For this review, take the finished solid that the model builds, in its own axes (mm). Face numbers are marked on the shaded views. A direction names the side the tool comes from. Give positions to 0.01 mm unless a question says otherwise; leave off trailing zeros. Order: outer loops, then holes, each group sorted by start corner. A loop starts at its lowest first (then second) coordinate and runs counter-clockwise, first axis right, second up. Notation, with made-up numbers: M -39,-32.75 L -16,-32.75 A14 cw -16,-5.75 Z; hole C 1,79 d9. An arc over 180 degrees is marked long. Use CSV: the item, a comma, the result in double quotes. Start each with the question number.
(1) Draft analysis for pull direction Y (two halves, no side actions). For the marked faces 1, 2 and 3, state which applies: pulls with the +Y half, pulls with the -Y half, needs draft (parallel to the pull), parting line crosses it, or undercut.
(2) Clearance check with flat-ended pins moving along their axes: P1, Ø1, axis at x = 2, z = 0.5, coming from the -Y side; P2, Ø4, axis at x = 0, y = 0, coming from the +Z side. State where each tip first meets the part, or that it passes through.
(3) Consider section C-C (z = 0.4). Write out the cut boundary in (x, y), and give its area (3 significant figures).
(4) Tool access review of the marked faces 4 and 5: name each direction out of +Z, -Z, +X, -X, +Y, -Y from which nothing blocks a thin tool from reaching the whole face with its end or side.
(5) Consider section D-D (z = 1.6). Write out the cut boundary in (x, y), and give its area (3 significant figures).
(6) Wall thickness on L1, parallel to Y at x = 0, z = 1; L2, parallel to Y at x = 0, z = 0.55; L3, parallel to Z at x = -1.25, y = -4: over which ranges is each line inside the solid? List them lowest first. Write a range as from..to.
(7) Consider section A-A (y = 0). Write out the cut boundary in (x, z), and give its area (3 significant figures).
```python
from build123d import *

# Parameters (mm, degrees)
F0_R     = 4
F1_DEPTH = 2
F0_R_2   = 4.6
F2_DEPTH = 0.6
F3_D     = 5
F4_SIZE  = 0.1


with BuildPart() as f1:
    # F0 (on Top) → F1 (new body)
    with BuildSketch(Plane.XY):
        Circle(F0_R)
    extrude(amount=F1_DEPTH)

    # F0 (on Top) → F2 (join)
    with BuildSketch(Plane.XY):
        Circle(F0_R_2)
        Circle(F0_R, mode=Mode.SUBTRACT)
    extrude(amount=F2_DEPTH)

    # F3 (through all)
    with Locations(Plane(origin=(0, 0, 0), x_dir=(1, 0, 0), z_dir=(0, 0, -1))):
        with Locations((0, 0)):
            Hole(F3_D / 2)

    # F4
    f4_edges = [f1.edges().sort_by_distance(p)[0] for p in [
        (-4, 0, 2),
        (-2.5, 0, 2),
        (-2.5, 0, 0),
    ]]
    chamfer(f4_edges, length=F4_SIZE)


solid = f1.part
```
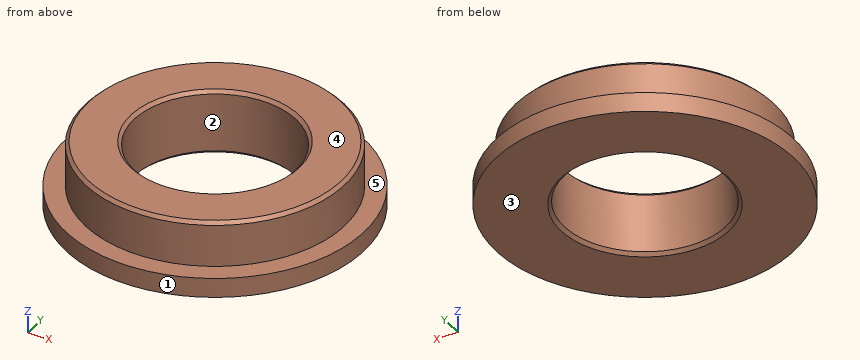
Check result:
1,face 1,"parting line crosses it"
1,face 2,"undercut"
1,face 3,"needs draft"
2,P1,"stops at y = -4.35"
2,P2,"passes through"
3,outline,"C 0,0 d9.2; hole C 0,0 d5"
3,area,"46.8 mm^2"
4,face 4,"+Z, +X, -X, +Y, -Y"
4,face 5,"+Z"
5,outline,"C 0,0 d8; hole C 0,0 d5"
5,area,"30.6 mm^2"
6,L1,"y = -4..-2.5, 2.5..4"
6,L2,"y = -4.6..-2.5, 2.5..4.6"
6,L3,"z = 0..0.6"
7,outline,"M -4.6,0 L -2.6,0 L -2.5,0.1 L -2.5,1.9 L -2.6,2 L -3.9,2 L -4,1.9 L -4,0.6 L -4.6,0.6 Z; M 2.5,0.1 L 2.6,0 L 4.6,0 L 4.6,0.6 L 4,0.6 L 4,1.9 L 3.9,2 L 2.6,2 L 2.5,1.9 Z"
7,area,"6.69 mm^2"
